Here's how the part is built. I have some questions about the finished solid (model axes, mm). A direction names the side the tool comes from. Give positions to 0.01 mm unless a question says otherwise; leave off trailing zeros. Write each loop counter-clockwise with the first axis right and the second up, starting at its lowest first coordinate (ties: lowest second). Pieces come first, ordered by that corner, then holes. Notation, with made-up numbers: (-16, 76) - (34, 76) arc R27 ccw to (34, 115) - close; hole circle Ø2 at (38, 56). An arc over 180 degrees is marked (long way). Use a Markdown table: item, result.
```python
from build123d import *

# Parameters (mm, degrees)
BOSS_EXTRUDE1_DEPTH       = 10.425440853
BOSS_EXTRUDE1_DEPTH_BACK  = 2
SKETCH1_R                 = 45
F_8_0MM_DOWEL_HOLE1_D     = 15
F_8_0MM_DOWEL_HOLE1_DEPTH = 7.425440853
F_8_0MM_DOWEL_HOLE1_TIP   = 7.5
F_3_0_3_DIAMETER_HOLE1_D  = 3


with BuildPart() as part:
    # Sketch1 → Boss-Extrude1 (new, two sides: drawn at the far end of the back side and taken through both)
    with BuildSketch(Plane(origin=(0, 0, 0), x_dir=(1, 0, 0), z_dir=(0, 1, 0)).offset(-BOSS_EXTRUDE1_DEPTH_BACK)):
        with Locations(Location((0, 0, 0), (0, 0, 270))):
            Circle(SKETCH1_R)
    extrude(amount=BOSS_EXTRUDE1_DEPTH + BOSS_EXTRUDE1_DEPTH_BACK)

    # Ø8.0mm Dowel Hole1
    with Locations(Plane(origin=(0, 10.425440853, 0), x_dir=(1, 0, 0), z_dir=(0, 1, 0))):
        with Locations((-16.606971943, 28.764119165), (-16.606971943, -28.764119165), (33.213943886, 0), (16.606971943, 28.764119165), (16.606971943, -28.764119165), (-33.213943886, 0)):
            Hole(F_8_0MM_DOWEL_HOLE1_D / 2, depth=F_8_0MM_DOWEL_HOLE1_DEPTH)
            with Locations((0, 0, -(F_8_0MM_DOWEL_HOLE1_DEPTH + F_8_0MM_DOWEL_HOLE1_TIP / 2))):  # 90° drill point
                Cone(0, F_8_0MM_DOWEL_HOLE1_D / 2, F_8_0MM_DOWEL_HOLE1_TIP, mode=Mode.SUBTRACT)

    # Ø3.0 (3) Diameter Hole1 (through all)
    with Locations(Plane(origin=(0, 10.425440853, 0), x_dir=(1, 0, 0), z_dir=(0, 1, 0))):
        with Locations((-34.641016151, 20), (0, -40), (34.641016151, 20)):
            Hole(F_3_0_3_DIAMETER_HOLE1_D / 2)


solid = part.part
```
Item 1: I need wall thicknesses on line 1 along X through (y, z) = (4.5, 35.5); line 2 along X through (y, z) = (3.25, 26.5); line 3 along Z through (x, y) = (-22, 3.75). Which ranges of each line are inside material? Lowest first, please. Write a range as [from, to].
Values:
| item | result |
|---|---|
| line 1 | x = [-27.65, -19.91], [-13.31, 13.31], [19.91, 27.65] |
| line 2 | x = [-36.37, -23.76], [-9.46, 9.46], [23.76, 36.37] |
| line 3 | z = [-39.26, -33.98], [-23.55, 23.55], [33.98, 39.26] |
Item 2: For faces 5 (the flat face through (1, -2, -1)), 6 (the cylindrical face through (22.56, 6.66, -24.2)), which set-ups out of +Z, -Z, +X, -X, +Y, -Y let a thin tool reach every point of the face, with its end or its side?
Values:
| item | result |
|---|---|
| face 5 | +Z, -Z, +X, -X, -Y |
| face 6 | +Y |
Item 3: Thinking about a two-plate mould opening in X: for faces 1 (the cylindrical face through (-17.235, 4.126, 41.569)), 2 (the flat face through (1, 10.425, -1)), 3 (the conical face through (35.9, -1.7, -0.8)), 4 (the cylindrical face through (17.583, 6.661, 21.328)), which applies, +X half, -X half, draft (parallel to the pull), parting line (faces both ways), or undercut?
Values:
| item | result |
|---|---|
| face 1 | parting line |
| face 2 | draft |
| face 3 | undercut |
| face 4 | undercut |
Item 4: If we section it at A-A, the plane x = 0: Write out the boundary of the cut face in (y, z).
Values:
| item | result |
|---|---|
| outline | (-2, -45) - (10.43, -45) - (10.43, 38.5) - (-2, 38.5) - close; (-2, 41.5) - (10.43, 41.5) - (10.43, 45) - (-2, 45) - close |
Item 5: If we section it at D-D, the plane y = 5: Count the separate pieces of the cut face and the enclosed holes in it, plus the area to 3 significant figures.
Values:
| item | result |
|---|---|
| separate pieces | 1 |
| enclosed holes | 9 |
| area | 5,280 mm2 |
Item 6: If we section it at B-B, the plane z = 40: Write out the boundary of the cut face in (x, y), plus the area to 3 significant figures.
Values:
| item | result |
|---|---|
| outline | (-20.62, -2) - (-1.5, -2) - (-1.5, 10.43) - (-20.62, 10.43) - close; (1.5, -2) - (20.62, -2) - (20.62, 10.43) - (1.5, 10.43) - close |
| area | 475 mm2 |
Item 7: If we section it at C-C, the plane z = -20: Write out the boundary of the cut face in (x, y), plus the area to 3 significant figures.
Values:
| item | result |
|---|---|
| outline | (-40.31, -2) - (-36.14, -2) - (-36.14, 10.43) - (-40.31, 10.43) - close; (-33.14, -2) - (33.14, -2) - (33.14, 10.43) - (-33.14, 10.43) - close; (36.14, -2) - (40.31, -2) - (40.31, 10.43) - (36.14, 10.43) - close |
| area | 927 mm2 |
Item 8: Will these pins go through, and if not, where does the flat tip stop? pin 1 Ø3 at (x, z) = (33, 33) entering from +Y; pin 2 Ø13.5 at (x, z) = (33.21, 0) entering from +Y; pin 3 Ø12 at (x, z) = (-16.61, -28.76) entering from +Y; pin 4 Ø1 at (y, z) = (6.5, 31) entering from -X.
Values:
| item | result |
|---|---|
| pin 1 | passes through |
| pin 2 | stops at y = 2.25 |
| pin 3 | stops at y = 1.51 |
| pin 4 | stops at x = -33.09 |
